CAD build for the part. Positions are in the model's coordinates, mm. Face numbers are marked on the shaded views. A direction names the side the tool comes from. Coordinates: 2 decimals unless noted, no trailing zeros. Write each loop counter-clockwise with the first axis right and the second up, starting at its lowest first coordinate (ties: lowest second). Pieces come first, ordered by that corner, then holes. Notation, with made-up numbers: (27.5, 62) - (49.5, 62) arc R8 cw to (49.5, 73) - close; hole circle Ø7 at (39.5, 75.5). An arc over 180 degrees is marked (long way). Answer in a Markdown table with one row per item. Add a question column.
Q1. 3-axis set-ups, long thin cutter, end or side, ignore diameter. For the marked faces 1, 2 and 3: which of +Z, -Z, +X, -X, +Y, -Y reach the whole face in a straight line?
Q2. Band-saw the part on B-B (z = -1.25). List the corners of the cut face in (x, y), and give its area (3 significant figures).
Q3. Pin check, flat tips, straight feed: pin 1 (1.5 mm diameter, centred on x = 10, z = 10.5, fed in from +Y); pin 2 (3 mm diameter, centred on x = -6.5, z = -5, fed in from -Y); pin 3 (1.5 mm diameter, centred on x = -5, z = 3.5, fed in from -Y); pin 4 (5 mm diameter, centred on x = 1.5, y = 13, fed in from +Z). Stop position of each tip, or through.
Q4. Drill centre lines: line 1 along Z through (x, y) = (10, 0.9); line 2 along Y through (x, z) = (-2.75, -1.5); line 3 along Y through (x, z) = (6.5, -10.5). Where is each one in solid material? Low to high. Write a range as from..to.
Q5. Band-saw the part on D-D (y = 10.5). List the corners of the cut face in (x, z), and give its area (3 significant figures).
Q6. Two-plate mould, pull along Y, no slides. Class the marked faces 4, 5 and 6: +Y half, -Y half, draft (parallel to the pull), parting line (faces both ways), or undercut.
Q7. Band-saw the part on A-A (x = 5.25). List the corners of the cut face in (y, z).
Q8. Band-saw the part on C-C (z = 11). List the corners of the cut face in (x, y), and give its area (3 significant figures).
Autodesk Inventor part; units mm, degrees
ref_plane "YZ Plane" through (0, 0, 0) normal (1, 0, 0) x (0, 1, 0)
ref_plane "XZ Plane" through (0, 0, 0) normal (0, 1, 0) x (-1, 0, 0)
ref_plane "XY Plane" through (0, 0, 0) normal (0, 0, 1) x (1, 0, 0)
sketch "Sketch1" plane through (0, 0, 0) normal (0, 1, 0) x (-1, 0, 0)
  line L0 (12, -12.5) -> (-12, -12.5)
  line L1 (-12, -12.5) -> (-12, 12.5)
  line L2 (-12, 12.5) -> (12, 12.5)
  line L3 (12, 12.5) -> (12, -12.5)
  line L4 (12, -12.5) -> (-12, 12.5) construction
  line L5 (-12, -12.5) -> (12, 12.5) construction
  circle A0 centre (2, 10.5) radius 1.25
  circle A1 centre (-10, 10.5) radius 1.25
  circle A2 centre (2, -10.5) radius 1.25
  circle A3 centre (-10, -10.5) radius 1.25
  line L6 (12, 0) -> (-12, 0) construction
  line L7 (10.1, -8.3) -> (11.8, -8.3)
  line L8 (11.8, -8.3) -> (11.8, 8.3)
  line L9 (11.8, 8.3) -> (10.1, 8.3)
  line L10 (10.1, 8.3) -> (10.1, -8.3)
  line L11 (10.1, -8.3) -> (11.8, 8.3) construction
  line L12 (11.8, -8.3) -> (10.1, 8.3) construction
  line L13 (6.6, -7.8) -> (10.1, -7.8)
  line L14 (10.1, -7.8) -> (10.1, 7.8)
  line L15 (10.1, 7.8) -> (6.6, 7.8)
  line L16 (6.6, 7.8) -> (6.6, -7.8)
  line L17 (6.6, -7.8) -> (10.1, 7.8) construction
  line L18 (10.1, -7.8) -> (6.6, 7.8) construction
  line L19 (1.5, -6.55) -> (-12, -6.55)
  line L20 (-12, -6.55) -> (-12, 6.55)
  line L21 (-12, 6.55) -> (1.5, 6.55)
  line L22 (1.5, 6.55) -> (1.5, -6.55)
  line L23 (1.5, -6.55) -> (-12, 6.55) construction
  line L24 (-12, -6.55) -> (1.5, 6.55) construction
  circle A4 centre (-5.25, 0) radius 6.75
  line L25 (-5.25, 6.55) -> (-5.25, -6.55) construction
  line L26 (-3.25, 8.55) -> (-3.25, -6.55)
  line L27 (-7.25, -8.55) -> (-7.25, 8.55)
  circle A5 centre (-5.25, 8.55) radius 2
  circle A6 centre (-5.25, -8.55) radius 2
  line L28 (-3.25, -8.55) -> (-3.25, -6.55)
  circle A7 centre (-5.25, 0) radius 6
  circle A8 centre (-5.25, 0) radius 5.5
  circle A9 centre (-5.25, 0) radius 8.7
  point P0 (0, 0)
  point P1 (10.95, 0)
  point P2 (8.35, 0)
  point P3 (-12, 5.4889)
  point P4 (-12, -5.4889)
  point P5 (-10.976, -6.55)
  point P6 (-7.25, -8.467)
  point P7 (-3.25, -8.467)
  point P8 (0.476, -6.55)
  point P9 (0.476, 6.55)
  point P10 (-3.25, 8.467)
  point P11 (-7.25, 8.467)
  point P12 (-10.976, 6.55)
  point P13 (12, -8.3)
  dimension "d0" = 25
  dimension "d1" = 24
  dimension "d2" = 2.5
  dimension "d3" = 21
  dimension "d4" = 12
  dimension "d5" = 2
  dimension "d6" = 16.6
  dimension "d7" = 1.7
  dimension "d8" = 15.6
  dimension "d9" = 3.5
  dimension "d10" = 13.5
  dimension "d11" = 13.1
  dimension "d12" = 4
  dimension "d13" = 4
  dimension "d14" = 11
  dimension "d15" = 12
  dimension "d16" = 17.4
  dimension "d35" = 0.2
  dimension "d36" = 4.75
  dimension "d37" = 10.5
extrude "Extrusion1" add sketch "Sketch1" along normal blind 1.6 contours L0 L1 L19 A9 L27 A6 L22 L21 L26 A5 L2 L3 | L1 A9 L19 | L1 A4 L27 L19 A9 | L19 L27 A9 | L21 A9 L1 | L1 A9 L21 L27 A4 | A4 L27 A7 | L27 A4 L19 | L19 A4 A6 L27 | A9 A6 L27 | A6 A4 A9 | A9 L27 L21 | L27 L21 A4 | A4 L21 L26 A7 L27 | L27 A7 L26 A4 L19 | L19 A6 A4 | A6 A4 | A6 A4 L19 L28 | L28 L19 A9 | L27 A5 A4 L21 | A9 A5 A4 | L27 A5 L26 A9 | A4 A5 L21 | A7 L26 A8 L27 | L27 A8 A7 | L27 A8 L26 A7 | L19 A4 A6 | L26 A4 L22 A9 L19 | L19 A4 L26 | A9 L22 L19 | A4 A5 | A9 L21 L26 | L26 L21 A4 A5 | A5 A4 L21 | A8 L26 L27 | L27 A8 | A7 L26 A8 | L26 A4 A7 | L22 A9 | L26 A4 L21 | L21 A9 L22 A4 L26 | L21 L22 A9 | A8 L26 | L10 L9 L8 L7 | L13 L16 L15 L10
extrude "Extrusion2" add sketch "Sketch1" along normal blind 3.5 from surface at 1.6 contours L1 A9 L19 | L1 A4 L27 L19 A9 | L19 L27 A9 | L21 A9 L1 | L1 A9 L21 L27 A4 | A4 L27 A7 | L27 A4 L19 | L19 A4 A6 L27 | A9 A6 L27 | A6 A4 A9 | A9 L27 L21 | L27 L21 A4 | A4 L21 L26 A7 L27 | L27 A7 L26 A4 L19 | L19 A6 A4 | A6 A4 | A6 A4 L19 L28 | L28 L19 A9 | L27 A5 A4 L21 | A9 A5 A4 | L27 A5 L26 A9 | A4 A5 L21 | A7 L26 A8 L27 | L27 A8 A7 | L27 A8 L26 A7 | L19 A4 A6 | L26 A4 L22 A9 L19 | L19 A4 L26 | A9 L22 L19 | A4 A5 | A9 L21 L26 | L26 L21 A4 A5 | A5 A4 L21 | A8 L26 L27 | L27 A8 | A7 L26 A8 | L26 A4 A7 | L26 A4 L21 | L21 A9 L22 A4 L26 | L21 L22 A9 | A8 L26
extrude "Extrusion3" add sketch "Sketch1" along normal blind 8.5 from surface at 5.1 contours A4 L27 A7 | A4 L21 L26 A7 L27 | L27 A7 L26 A4 L19 | L19 A6 A4 | A6 A4 | A4 A5 L21 | A7 L26 A8 L27 | L27 A8 A7 | L27 A8 L26 A7 | L19 A4 A6 | A4 A5 | A5 A4 L21 | A8 L26 L27 | L27 A8 | A7 L26 A8 | L26 A4 A7 | A8 L26
extrude "Extrusion4" add sketch "Sketch1" along normal blind 3.2 from surface at 13.6 contours A8 L26 L27 | L27 A8 | A8 L26
extrude "Extrusion5" add sketch "Sketch1" along normal blind 2.8 from surface at 16.8 contours A7 L26 A8 L27 | L27 A8 A7 | L27 A8 L26 A7 | A8 L26 L27 | L27 A8 | A7 L26 A8 | A8 L26
extrude "Extrusion6" add sketch "Sketch1" along normal blind 4.5 from surface at 19.6 contours A9 L1 | L1 A4 L27 L19 A9 | L19 L27 A9 | L1 A9 L21 L27 A4 | A4 L27 A7 | L27 A4 L19 | L19 A4 A6 L27 | A6 A4 A9 | A9 L27 L21 | L27 L21 A4 | A4 L21 L26 A7 L27 | L27 A7 L26 A4 L19 | L19 A6 A4 | A6 A4 | A6 A4 L19 L28 | L28 L19 A9 | L27 A5 A4 L21 | A9 A5 A4 | A4 A5 L21 | A7 L26 A8 L27 | L27 A8 A7 | L27 A8 L26 A7 | L19 A4 A6 | L26 A4 L22 A9 L19 | L19 A4 L26 | A4 A5 | A9 L21 L26 | L26 L21 A4 A5 | A5 A4 L21 | A8 L26 L27 | L27 A8 | A7 L26 A8 | L26 A4 A7 | L22 A9 | L26 A4 L21 | L21 A9 L22 A4 L26 | A8 L26
extrude "Extrusion7" add sketch "Sketch1" against normal blind 2 contours L10 L9 L8 L7 | L13 L16 L15 L10
fillet "Fillet1" radius 2 4 edges at (-12, 0.8, -12.5) (-12, 0.8, 12.5) (12, 0.8, 12.5) (12, 0.8, -12.5)
sketch "Sketch2" plane through (0, 0, 0) normal (0, 0, 1) x (1, 0, 0)
  line L0 (-3.45, 24.1) -> (13.95, 24.1)
  line L1 (5.25, 24.1) -> (5.25, 0)
  line L2 (-10, 0) -> (10, 0)
  arc A0 (12.45, 24.1) -> (-1.95, 24.1) centre (5.25, -5.0232) ccw
  line L3 (12.45, 24.1) -> (-1.95, 24.1)
  line L4 (5.25, 24.1) -> (5.25, 24.9768)
  point P0 (0, 0)
  dimension "d32" = 1.5
  dimension "d33" = 30
revolve "Revolution1" add sketch "Sketch2" angle 360 about axis through (5.25, 24.1, 0) along (0, 1, 0) picked at (9.2588, 24.262) contours L4 A0 L0
sketch "Sketch3" plane through (0, 0, 0) normal (0, 0, 1) x (1, 0, 0)
  line L0 (-3.45, 24.1) -> (13.95, 24.1) construction
  line L1 (5.25, 24.1) -> (5.25, 38.8159)
  line L2 (5.25, 24.1) -> (119.5505, 34.1)
  line L3 (119.5505, 34.1) -> (5.25, 34.1) construction
  point P0 (0, 0)
  dimension "d38" = 85
  dimension "d41" = 10
properties part number "Arducam Camera"
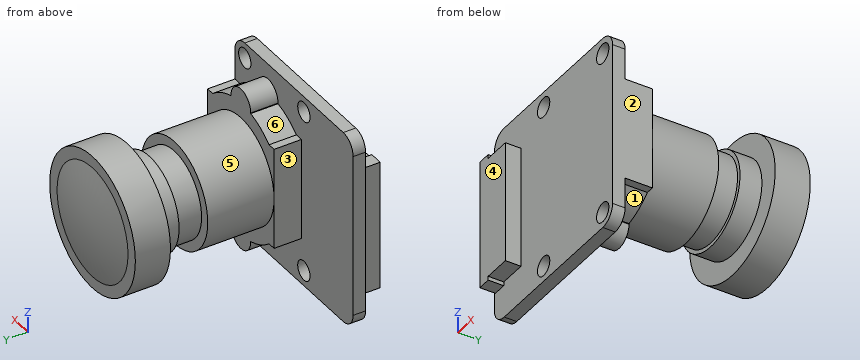
Checked values:
| question | item | result |
|---|---|---|
| 1 | face 1 | -Z, +X, +Y |
| 1 | face 2 | +Z, -Z, +X, -Y |
| 1 | face 3 | +Z, -Z, -X |
| 2 | outline | (-12, 0) - (-11.8, 0) - (-11.8, -2) - (-6.6, -2) - (-6.6, 0) - (12, 0) - (12, 5.1) - (11.88, 5.1) - (11.88, 13.6) - (10.61, 13.6) - (10.61, 16.8) - (11.12, 16.8) - (11.12, 19.6) - (13.86, 19.6) - (13.86, 24.1) - (12.34, 24.1) arc R29.97 ccw to (-1.84, 24.1) - (-3.36, 24.1) - (-3.36, 19.6) - (-0.62, 19.6) - (-0.62, 16.8) - (-0.11, 16.8) - (-0.11, 13.6) - (-1.38, 13.6) - (-1.38, 5.1) - (-1.5, 5.1) - (-1.5, 1.6) - (-12, 1.6) - close |
| 2 | area | 362 mm² |
| 3 | pin 1 | passes through |
| 3 | pin 2 | stops at y = -2 |
| 3 | pin 3 | stops at y = 0 |
| 3 | pin 4 | stops at z = 6.63 |
| 4 | line 1 | z = -12.5..-11.75, -9.25..9.25, 11.75..12.5 |
| 4 | line 2 | y = 0..1.6, 19.6..24.1 |
| 4 | line 3 | y = 0..1.6 |
| 5 | outline | circle Ø13.5 at (5.25, 0) |
| 5 | area | 143 mm² |
| 6 | face 4 | -Y half |
| 6 | face 5 | undercut |
| 6 | face 6 | draft |
| 7 | outline | (0, -12.5) - (1.6, -12.5) - (1.6, -10.55) - (5.1, -10.55) - (5.1, -6.75) - (13.6, -6.75) - (13.6, -5.5) - (16.8, -5.5) - (16.8, -6) - (19.6, -6) - (19.6, -8.7) - (24.1, -8.7) - (24.1, -7.2) arc R30 ccw to (24.1, 7.2) - (24.1, 8.7) - (19.6, 8.7) - (19.6, 6) - (16.8, 6) - (16.8, 5.5) - (13.6, 5.5) - (13.6, 6.75) - (5.1, 6.75) - (5.1, 10.55) - (1.6, 10.55) - (1.6, 12.5) - (0, 12.5) - close |
| 8 | outline | (-11.94, 0) - (-3.15, 0) - (-3.15, 1.6) - (-11.94, 1.6) - close; (-0.85, 0) - (8.85, 0) - (8.85, 1.6) - (-0.85, 1.6) - close; (11.15, 0) - (11.94, 0) - (11.94, 1.6) - (11.15, 1.6) - close |
| 8 | area | 30.9 mm² |
